The drawing under review shows one solid part. Ordinate dimensions are in mm from its lowest x, y, z. Give positions to 0.01 mm unless a question says otherwise; leave off trailing zeros. Order: outer loops, then holes, each group sorted by start corner. A loop starts at its lowest first (then second) coordinate and runs counter-clockwise, first axis right, second up. Notation, with made-up numbers: (-37.5, 32.5) - (-19.5, 32.5) arc R28 ccw to (-19.5, 69.5) - close; hole circle Ø1 at (87, -6). An arc over 180 degrees is marked (long way). Write item = value, one per line. Start each with the question number.
1. We need section D-D, the plane x = 62. Give the boundary of the cut face in (y, z) (1 decimal).
2. We need section C-C, the plane y = 90. Give the boundary of the cut face in (x, z) (1 decimal).
3. We need section A-A, the plane y = 72.39. Give the boundary of the cut face in (x, z) (1 decimal).
4. For P1, Ø1, axis at y = 40.5, z = 1, coming from the +X side; P2, Ø1, axis at x = 48, z = 1, coming from the +Y side, all flat-tipped, find the tip position at first contact; note any pin that passes through.
5. We need section B-B, the plane x = 12.7. Give the boundary of the cut face in (y, z) (1 decimal).
6. Wall thickness on probe 1 along Y at (x, z) = (12.7, 1.6) (1 decimal); probe 2 along X at (y, z) = (56, 1.35) (1 decimal); probe 3 along X at (y, z) = (10.5, 2.2): over which ranges is each line inside the solid? List them lowest first.
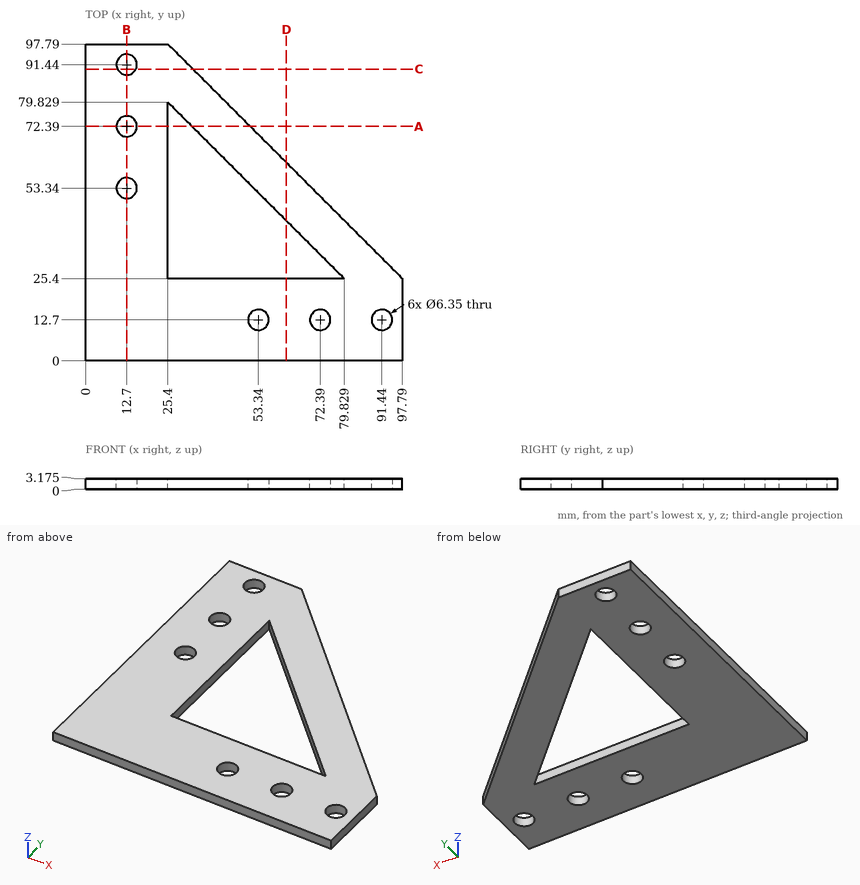
Model answer:
q1.outline = (0, 0) - (25.4, 0) - (25.4, 3.2) - (0, 3.2) - close; (43.2, 0) - (61.2, 0) - (61.2, 3.2) - (43.2, 3.2) - close
q2.outline = (0, 0) - (9.9, 0) - (9.9, 3.2) - (0, 3.2) - close; (15.5, 0) - (33.2, 0) - (33.2, 3.2) - (15.5, 3.2) - close
q3.outline = (0, 0) - (9.5, 0) - (9.5, 3.2) - (0, 3.2) - close; (15.9, 0) - (25.4, 0) - (25.4, 3.2) - (15.9, 3.2) - close; (32.8, 0) - (50.8, 0) - (50.8, 3.2) - (32.8, 3.2) - close
q4.P1 = 83.19
q4.P2 = 75.69
q5.outline = (0, 0) - (50.2, 0) - (50.2, 3.2) - (0, 3.2) - close; (56.5, 0) - (69.2, 0) - (69.2, 3.2) - (56.5, 3.2) - close; (75.6, 0) - (88.3, 0) - (88.3, 3.2) - (75.6, 3.2) - close; (94.6, 0) - (97.8, 0) - (97.8, 3.2) - (94.6, 3.2) - close
q6.probe_1 = 0 to 50.2, 56.5 to 69.2, 75.6 to 88.3, 94.6 to 97.8
q6.probe_2 = 0 to 11, 14.4 to 25.4, 49.2 to 67.2
q6.probe_3 = 0 to 51.05, 55.63 to 70.1, 74.68 to 89.15, 93.73 to 97.79
